```python
from build123d import *

# Parameters (mm, degrees)
SKETCH1_R           = 6
BOSS_EXTRUDE1_DEPTH = 155
SKETCH3_R           = 2
CUT_EXTRUDE1_DEPTH  = 10
CHAMFER1_SIZE       = 0.5
FILLET1_R           = 0.3


with BuildPart() as part:
    # Sketch1 → Boss-Extrude1 (new body)
    with BuildSketch(Plane(origin=(0, 0, 0), x_dir=(0, 0, -1), z_dir=(1, 0, 0))):
        Circle(SKETCH1_R)
    extrude(amount=BOSS_EXTRUDE1_DEPTH)

    # Sketch2 → Cut-Revolve1 (revolve, cut)
    with BuildSketch(Plane.XY):
        Polygon((0, 5), (0, 6), (9, 6), (9, 5), (4, 5), (4, 4.8), (2.9, 4.8), (2.9, 5), align=None)
    revolve(axis=Axis((155, 0, 0), (-1, 0, 0)), mode=Mode.SUBTRACT)

    # Sketch3 → Cut-Extrude1 (cut, symmetric)
    with BuildSketch(Plane(origin=(0, 0, 0), x_dir=(1, 0, 0), z_dir=(0, 1, 0))):
        with Locations((18.5, 0)):
            Circle(SKETCH3_R)
    extrude(amount=CUT_EXTRUDE1_DEPTH, both=True, mode=Mode.SUBTRACT)

    # Chamfer1
    chamfer1_edges = [part.edges().sort_by_distance(p)[0] for p in [
        (155, 0, 6),
        (0, -5, 0),
    ]]
    chamfer(chamfer1_edges, length=CHAMFER1_SIZE)

    # Fillet1
    fillet1_edges = [part.edges().sort_by_distance(p)[0] for p in [
        (9, -5, 0),
    ]]
    fillet(fillet1_edges, radius=FILLET1_R)


solid = part.part
```
Design review of the part built by this model. Coordinates are the model's own, in mm. A direction names the side the tool comes from. Coordinates: 2 decimals unless noted, no trailing zeros. Order: outer loops, then holes, each group sorted by start corner. A loop starts at its lowest first (then second) coordinate and runs counter-clockwise, first axis right, second up.
1) Take a section at C-C, the plane x = 28.5. Give the boundary of the cut face in (y, z).
2) Take a section at B-B, the plane y = 0. Give the boundary of the cut face in (x, z), and give its area (3 significant figures).
3) Wall thickness on line 1 along Y through (x, z) = (106, -0.5); line 2 along X through (y, z) = (-1, 0); line 3 along Z through (x, y) = (18.5, -0.25): over which ranges is each line inside the solid? List them lowest first.
4) Clearance check with flat-ended pins moving along their axes: pin 1 (3 mm diameter, centred on x = 49.5, y = 3, fed in from +Z); pin 2 (1.5 mm diameter, centred on x = 108.5, y = -2.5, fed in from +Z); pin 3 (3.5 mm diameter, centred on x = 18.5, z = 0, fed in from +Y); pin 4 (5 mm diameter, centred on x = 42.5, z = -4, fed in from -Y). State where each tip first meets the part, or that it passes through.
5) Mouldability with a two-part tool opening along Z and no side actions: class faces 4 (the cylindrical face through (16.9, 0.1, 1.2)), 5 (the flat face through (0, 0, 0)), 6 (the cylindrical face through (80.73, -2.3, -5.54)) as +Z half, -Z half, draft (parallel to the pull), parting line (faces both ways), or undercut.
6) Take a section at A-A, the plane z = 0. Give the boundary of the cut face in (x, y), and give its area (3 significant figures).
7) For faces 1 (the flat face through (155, 0, 0)), 2 (the cylindrical face through (3.44, 2.58, -4.05)), 3 (the cylindrical face through (1.68, -1.08, 4.88)), list the 3-axis set-ups (+Z, -Z, +X, -X, +Y, -Y) from which the entire face can be reached by the end or side of a thin tool; tool diameter is ignored.
Returned:
1. outline: circle Ø12 at (0, 0)
2. outline: (0, -4.5) - (0.5, -5) - (2.9, -5) - (2.9, -4.8) - (4, -4.8) - (4, -5) - (8.7, -5) arc R0.3 cw to (9, -5.3) - (9, -6) - (154.5, -6) - (155, -5.5) - (155, 5.5) - (154.5, 6) - (9, 6) - (9, 5.3) arc R0.3 cw to (8.7, 5) - (4, 5) - (4, 4.8) - (2.9, 4.8) - (2.9, 5) - (0.5, 5) - (0, 4.5) - close; hole circle Ø4 at (18.5, 0)
2. area: 1,830 mm2
3. line 1: y = -5.98 to 5.98
3. line 2: x = 0 to 16.5, 20.5 to 155
3. line 3: z = -5.99 to -2, 2 to 5.99
4. pin 1: stops at z = 5.81
4. pin 2: stops at z = 5.74
4. pin 3: passes through
4. pin 4: stops at y = -5.81
5. face 4: undercut
5. face 5: draft
5. face 6: parting line
6. outline: (0, -4.5) - (0.5, -5) - (2.9, -5) - (2.9, -4.8) - (4, -4.8) - (4, -5) - (8.7, -5) arc R0.3 cw to (9, -5.3) - (9, -6) - (16.5, -6) - (16.5, 6) - (9, 6) - (9, 5.3) arc R0.3 cw to (8.7, 5) - (4, 5) - (4, 4.8) - (2.9, 4.8) - (2.9, 5) - (0.5, 5) - (0, 4.5) - close; (20.5, -6) - (154.5, -6) - (155, -5.5) - (155, 5.5) - (154.5, 6) - (20.5, 6) - close
6. area: 1,790 mm2
7. face 1: +Z, -Z, +X, +Y, -Y
7. face 2: none
7. face 3: -X
